Drawing for the job (mm, zero at the part's lowest x, y, z). Round coordinates to 2 decimals unless told otherwise and drop trailing zeros. Loops run counter-clockwise (first coordinate to the right, second up) from the corner with the lowest first, then second, coordinate; pieces in that order, holes last. Notation, with made-up numbers: M 56,28 L 96,28 A25 ccw 96,48 Z; hole C 89,-8.75 d3. An arc over 180 degrees is marked long. Use a Markdown table: item, result. Add a question column.
Q1. Cut at B-B (z = 7.5). Give the cut face in (x, y).
Q2. Probe line 1 (Z direction, x = 112.5, y = 1.65); line 2 (X direction, y = 3.25, z = 52.5); line 3 (X direction, y = 3.1, z = 9.5). List the from-to ranges inside material, lowest first. Write a range as from..to.
Q3. Cut at D-D (y = 2.45). Give the cut face in (x, z).
Q4. Cut at A-A (x = 112.5). Give the cut face in (y, z).
Q5. Cut at C-C (z = 33). Give the cut face in (x, y).
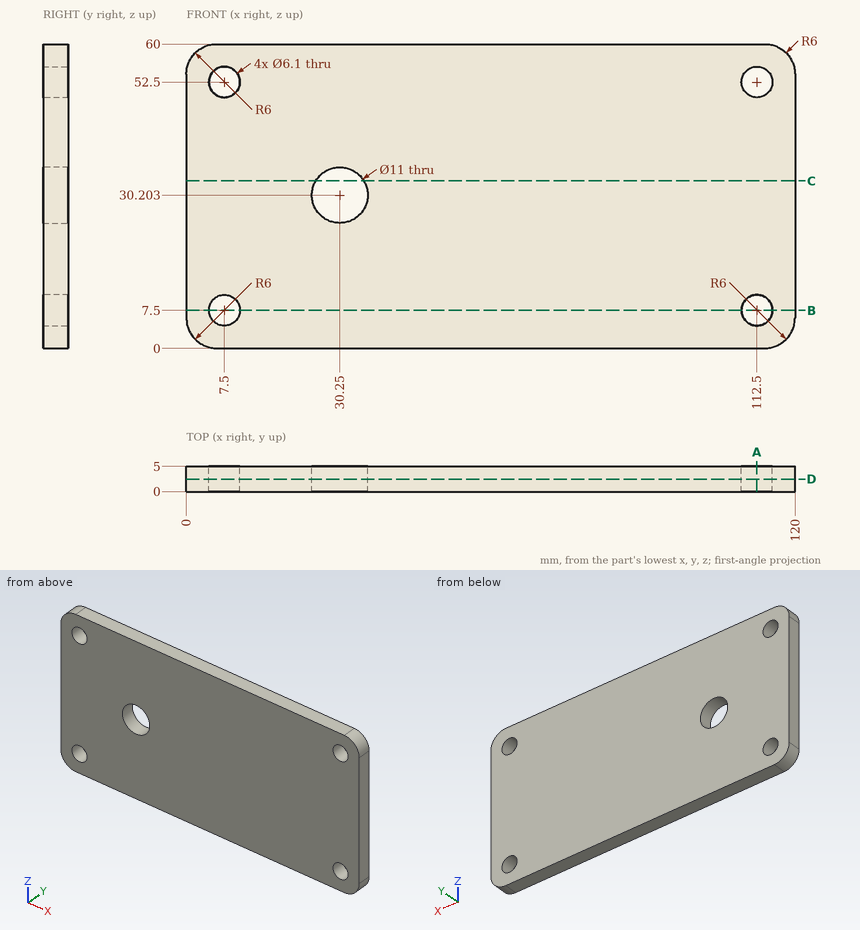
Checked values:
| question | item | result |
|---|---|---|
| 1 | outline | M 0,0 L 4.45,0 L 4.45,5 L 0,5 Z; M 10.55,0 L 109.45,0 L 109.45,5 L 10.55,5 Z; M 115.55,0 L 120,0 L 120,5 L 115.55,5 Z |
| 2 | line 1 | z = 0..4.45, 10.55..49.45, 55.55..60 |
| 2 | line 2 | x = 0..4.45, 10.55..109.45, 115.55..120 |
| 2 | line 3 | x = 0..5.2, 9.8..110.2, 114.8..120 |
| 3 | outline | M 0,6 A6 ccw 6,0 L 114,0 A6 ccw 120,6 L 120,54 A6 ccw 114,60 L 6,60 A6 ccw 0,54 Z; hole C 7.5,7.5 d6.1; hole C 7.5,52.5 d6.1; hole C 30.25,30.2 d11; hole C 112.5,7.5 d6.1; hole C 112.5,52.5 d6.1 |
| 4 | outline | M 0,0 L 5,0 L 5,4.45 L 0,4.45 Z; M 0,10.55 L 5,10.55 L 5,49.45 L 0,49.45 Z; M 0,55.55 L 5,55.55 L 5,60 L 0,60 Z |
| 5 | outline | M 0,0 L 25.51,0 L 25.51,5 L 0,5 Z; M 34.99,0 L 120,0 L 120,5 L 34.99,5 Z |
